from build123d import *

# Parameters (mm, degrees)
CROQUIS1_R              = 2.5
CROQUIS1_R_2            = 2
SALIENTE_EXTRUIR1_DEPTH = 3
CROQUIS2_W              = 20
CROQUIS2_H              = 75
CORTAR_EXTRUIR1_DEPTH   = 10
CROQUIS3_W              = 35
CROQUIS3_H              = 15
CORTAR_EXTRUIR2_DEPTH   = 10
CROQUIS4_R              = 1.5
CORTAR_EXTRUIR3_DEPTH   = 10
CROQUIS5_R              = 1.5
CORTAR_EXTRUIR4_DEPTH   = 10
CORTAR_EXTRUIR5_DEPTH   = 10


with BuildPart() as part:
    # Croquis1 → Saliente-Extruir1 (new body)
    with BuildSketch(Plane(origin=(0, 0, 0), x_dir=(1, 0, 0), z_dir=(0, 1, 0))):
        with BuildLine():
            Line((-20, 0), (-140, 0))
            ThreePointArc((-140, 0), (-154.142135624, -5.857864376), (-160, -20))
            Line((-160, -20), (-160, -90))
            Line((-160, -90), (0, -90))
            Line((0, -90), (0, -20))
            ThreePointArc((0, -20), (-5.857864376, -5.857864376), (-20, 0))
        make_face()
        with Locations(Location((-101.245, -83, 0), (0, 0, 270))):
            Circle(CROQUIS1_R, mode=Mode.SUBTRACT)
        with Locations(Location((-58.755, -83, 0), (0, 0, 270))):
            Circle(CROQUIS1_R, mode=Mode.SUBTRACT)
        with Locations(Location((-132.5, -25, 0), (0, 0, 270))):
            Circle(CROQUIS1_R_2, mode=Mode.SUBTRACT)
        with Locations(Location((-107.5, -25, 0), (0, 0, 270))):
            Circle(CROQUIS1_R_2, mode=Mode.SUBTRACT)
        with Locations(Location((-107.5, -51, 0), (0, 0, 270))):
            Circle(CROQUIS1_R_2, mode=Mode.SUBTRACT)
        with Locations(Location((-132.5, -51, 0), (0, 0, 270))):
            Circle(CROQUIS1_R_2, mode=Mode.SUBTRACT)
        with Locations(Location((-52.5, -25, 0), (0, 0, 270))):
            Circle(CROQUIS1_R_2, mode=Mode.SUBTRACT)
        with Locations(Location((-27.5, -25, 0), (0, 0, 270))):
            Circle(CROQUIS1_R_2, mode=Mode.SUBTRACT)
        with Locations(Location((-52.5, -51, 0), (0, 0, 270))):
            Circle(CROQUIS1_R_2, mode=Mode.SUBTRACT)
        with Locations(Location((-27.5, -51, 0), (0, 0, 270))):
            Circle(CROQUIS1_R_2, mode=Mode.SUBTRACT)
    extrude(amount=SALIENTE_EXTRUIR1_DEPTH)

    # Croquis2 → Cortar-Extruir1 (cut)
    with BuildSketch(Plane.XZ):
        with Locations((-150, 37.5)):
            Rectangle(CROQUIS2_W, CROQUIS2_H)
        with Locations((-10, 37.5)):
            Rectangle(CROQUIS2_W, CROQUIS2_H)
    extrude(amount=-CORTAR_EXTRUIR1_DEPTH, mode=Mode.SUBTRACT)

    # Croquis3 → Cortar-Extruir2 (cut)
    with BuildSketch(Plane.XZ):
        with Locations((-80, 82.5)):
            Rectangle(CROQUIS3_W, CROQUIS3_H)
    extrude(amount=-CORTAR_EXTRUIR2_DEPTH, mode=Mode.SUBTRACT)

    # Croquis4 → Cortar-Extruir3 (cut)
    with BuildSketch(Plane(origin=(0, 3, 0), x_dir=(1, 0, 0), z_dir=(0, 1, 0))):
        with Locations(Location((-30.71, -63.73, 0), (0, 0, 270))):
            Circle(CROQUIS4_R)
        with Locations(Location((-30.71, -75.73, 0), (0, 0, 270))):
            Circle(CROQUIS4_R)
        with Locations(Location((-30.71, -87.73, 0), (0, 0, 270))):
            Circle(CROQUIS4_R)
        with Locations(Location((-129.29, -63.73, 0), (0, 0, 270))):
            Circle(CROQUIS4_R)
        with Locations(Location((-129.29, -75.73, 0), (0, 0, 270))):
            Circle(CROQUIS4_R)
        with Locations(Location((-129.29, -87.73, 0), (0, 0, 270))):
            Circle(CROQUIS4_R)
    extrude(amount=-CORTAR_EXTRUIR3_DEPTH, mode=Mode.SUBTRACT)

    # Croquis5 → Cortar-Extruir4 (cut)
    with BuildSketch(Plane.XZ):
        with Locations(Location((-130, 3, 0), (0, 0, 270))):
            Circle(CROQUIS5_R)
        with Locations(Location((-110, 3, 0), (0, 0, 270))):
            Circle(CROQUIS5_R)
        with Locations(Location((-90, 3, 0), (0, 0, 270))):
            Circle(CROQUIS5_R)
        with Locations(Location((-70, 3, 0), (0, 0, 270))):
            Circle(CROQUIS5_R)
        with Locations(Location((-50, 3, 0), (0, 0, 270))):
            Circle(CROQUIS5_R)
        with Locations(Location((-30, 3, 0), (0, 0, 270))):
            Circle(CROQUIS5_R)
        with Locations(Location((-157, 86, 0), (0, 0, 270))):
            Circle(CROQUIS5_R)
        with Locations(Location((-157, 78, 0), (0, 0, 270))):
            Circle(CROQUIS5_R)
        with Locations(Location((-3, 86, 0), (0, 0, 270))):
            Circle(CROQUIS5_R)
        with Locations(Location((-3, 78, 0), (0, 0, 270))):
            Circle(CROQUIS5_R)
    extrude(amount=-CORTAR_EXTRUIR4_DEPTH, mode=Mode.SUBTRACT)

    # Croquis6 → Cortar-Extruir5 (cut)
    with BuildSketch(Plane(origin=(0, 0, 0), x_dir=(-1, 0, 0), z_dir=(0, -1, 0))):
        with BuildLine():
            Line((64.522468013, -52), (60.522468013, -52))
            ThreePointArc((60.522468013, -52), (57.694040888, -50.828427125), (56.522468013, -48))
            Line((56.522468013, -48), (56.522468013, -25))
            ThreePointArc((56.522468013, -25), (57.694040888, -22.171572875), (60.522468013, -21))
            Line((60.522468013, -21), (64.522468013, -21))
            ThreePointArc((64.522468013, -21), (67.350895137, -22.171572875), (68.522468013, -25))
            Line((68.522468013, -25), (68.522468013, -48))
            ThreePointArc((68.522468013, -48), (67.350895137, -50.828427125), (64.522468013, -52))
        make_face()
        with BuildLine():
            Line((96.522468013, -52), (92.522468013, -52))
            ThreePointArc((92.522468013, -52), (89.694040888, -50.828427125), (88.522468013, -48))
            Line((88.522468013, -48), (88.522468013, -25))
            ThreePointArc((88.522468013, -25), (89.694040888, -22.171572875), (92.522468013, -21))
            Line((92.522468013, -21), (96.522468013, -21))
            ThreePointArc((96.522468013, -21), (99.350895137, -22.171572875), (100.522468013, -25))
            Line((100.522468013, -25), (100.522468013, -48))
            ThreePointArc((100.522468013, -48), (99.350895137, -50.828427125), (96.522468013, -52))
        make_face()
    extrude(amount=-CORTAR_EXTRUIR5_DEPTH, mode=Mode.SUBTRACT)


solid = part.part
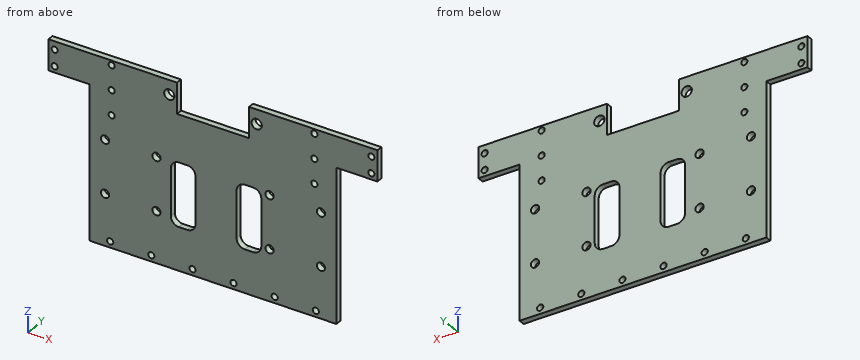
Verification items for the finished model (mm, model axes). Give positions to 0.01 mm unless a question says otherwise; leave off trailing zeros. Write each loop counter-clockwise with the first axis right and the second up, starting at its lowest first coordinate (ties: lowest second). Pieces come first, ordered by that corner, then holes. Notation, with made-up numbers: M 59,53.5 L 72,53.5 A22 cw 72,79.5 Z; hole C 65,78.25 d7. An arc over 180 degrees is marked long. Put each result on its own line as item: value. Start each with the question number.
1. Scan lines: line 1 along Z through (x, y) = (-157, 1.2); line 2 along Z through (x, y) = (-132.5, 2.2); line 3 along X through (y, z) = (0.7, 83) (3 decimals). Record each from-to range of solid material in increasing order. Write a range as [from, to].
2. Go/stop test with flat-tipped pins: pin 1 Ø1.5 at (y, z) = (1, 68) entering from -X; pin 2 Ø1 at (y, z) = (0.5, 73.5) entering from +X; pin 3 Ø1.8 at (x, z) = (-90, 3) entering from -Y (3 decimals); pin 4 Ø1.5 at (x, y) = (-88, 2) entering from +Z. Record where each tip stops, or that it passes through.
3. Section check D-D (x = -74). Record the cut outline in (y, z).
4. Section check A-A (x = -157). Record the cut outline in (y, z), and give its area (3 significant figures).
5. Section check B-B (z = 63.73). Record the cut outline in (x, y).
6. Section check C-C (z = 3). Record the cut outline in (x, y), and give its area (3 significant figures).
Answer list:
1. line 1: [75, 76.5], [79.5, 84.5], [87.5, 90]
1. line 2: [0, 23], [27, 49], [53, 90]
1. line 3: [-160, -103.745], [-98.745, -97.5], [-62.5, -61.255], [-56.255, 0]
2. pin 1: x = -140
2. pin 2: x = -20
2. pin 3: through
2. pin 4: z = 75
3. outline: M 0,0 L 3,0 L 3,75 L 0,75 Z
4. outline: M 0,75 L 3,75 L 3,76.5 L 0,76.5 Z; M 0,79.5 L 3,79.5 L 3,84.5 L 0,84.5 Z; M 0,87.5 L 3,87.5 L 3,90 L 0,90 Z
4. area: 27.0 mm2
5. outline: M -140,0 L -130.79,0 L -130.79,3 L -140,3 Z; M -127.79,0 L -32.21,0 L -32.21,3 L -127.79,3 Z; M -29.21,0 L -20,0 L -20,3 L -29.21,3 Z
6. outline: M -140,0 L -131.5,0 L -131.5,3 L -140,3 Z; M -128.5,0 L -111.5,0 L -111.5,3 L -128.5,3 Z; M -108.5,0 L -91.5,0 L -91.5,3 L -108.5,3 Z; M -88.5,0 L -71.5,0 L -71.5,3 L -88.5,3 Z; M -68.5,0 L -51.5,0 L -51.5,3 L -68.5,3 Z; M -48.5,0 L -31.5,0 L -31.5,3 L -48.5,3 Z; M -28.5,0 L -20,0 L -20,3 L -28.5,3 Z
6. area: 306 mm2
